from build123d import *

# Parameters (mm, degrees)
EXTRUDE_2_DEPTH                 = 50
SKETCH_4_W                      = 120
SKETCH_4_H                      = 97.901728648
CUT_EXTRUDE_1_DEPTH             = 50
PATTERN_CIRCULAR_1_COUNT        = 8
EXTRUDE_3_DEPTH                 = 50
CUT_EXTRUDE_2_REACH             = 100.489
CUT_EXTRUDE_2_DIRECTION_2_REACH = 100.489
PATTERN_CIRCULAR_3_COUNT        = 8
EXTRUDE_4_DEPTH                 = 50


with BuildPart() as part:
    # Sketch 3 → Extrude 2 (new body)
    with BuildSketch(Plane(origin=(0, 0, 0), x_dir=(1, 0, 0), z_dir=(0, 1, 0))):
        Polygon((-60, 0), (-42.426406871, -42.426406871), (0, -60), (42.426406871, -42.426406871), (60, 0), (42.426406871, 42.426406871), (0, 60), (-42.426406871, 42.426406871), align=None)
        Polygon((-11.480502971, -27.716385975), (11.480502971, -27.716385975), (27.716385975, -11.480502971), (27.716385975, 11.480502971), (11.480502971, 27.716385975), (-11.480502971, 27.716385975), (-27.716385975, 11.480502971), (-27.716385975, -11.480502971), align=None, mode=Mode.SUBTRACT)
    extrude(amount=EXTRUDE_2_DEPTH)

    # Sketch 4 → Cut-Extrude 1 (cut)
    with BuildSketch(Plane(origin=(-16.852857596, 22.400493343, 40.686397374), x_dir=(0.9400294128280147, 0.16450882670917247, 0.2988001823175307), z_dir=(-0.3410933933957357, 0.4533747611963636, 0.8234722963718466))):
        Rectangle(SKETCH_4_W, SKETCH_4_H)
    cut_extrude_1 = extrude(amount=CUT_EXTRUDE_1_DEPTH, mode=Mode.SUBTRACT)

    # Pattern Circular 1: Cut-Extrude 1 ×8 about axis
    pattern_circular_1_axis = Axis((0, 0, 0), (0, 1, 0))
    for i in range(1, PATTERN_CIRCULAR_1_COUNT):
        add(cut_extrude_1.rotate(pattern_circular_1_axis, i * 360 / PATTERN_CIRCULAR_1_COUNT), mode=Mode.SUBTRACT)

    # Sketch 5 → Extrude 3 (add)
    with BuildSketch(Plane(origin=(0, 0, 0), x_dir=(1, 0, 0), z_dir=(0, 1, 0))):
        Polygon((-27.716385975, 11.480502971), (-60, 0), (-27.716385975, -11.480502971), align=None)
    extrude_3 = extrude(amount=EXTRUDE_3_DEPTH)

    # Sketch 6 → Cut-Extrude 2 (cut, up to next)
    with BuildSketch(Plane.XY, mode=Mode.PRIVATE) as cut_extrude_2_sk1:
        Polygon((-27.716385975, 50), (-60, 50), (-60, 25), align=None)
    cut_extrude_2_tool1 = extrude(cut_extrude_2_sk1.sketch, amount=-CUT_EXTRUDE_2_REACH, mode=Mode.PRIVATE) & part.part
    cut_extrude_2 = cut_extrude_2_tool1.solids().sort_by_distance((-49.238795, 41.666667, 0))[0]
    add(cut_extrude_2, mode=Mode.SUBTRACT)

    # Sketch 6 → Cut-Extrude 2 direction 2 (cut, up to next)
    with BuildSketch(Plane.XY, mode=Mode.PRIVATE) as cut_extrude_2_direction_2_sk1:
        Polygon((-27.716385975, 50), (-60, 50), (-60, 25), align=None)
    cut_extrude_2_direction_2_tool1 = extrude(cut_extrude_2_direction_2_sk1.sketch, amount=CUT_EXTRUDE_2_DIRECTION_2_REACH, mode=Mode.PRIVATE) & part.part
    cut_extrude_2_direction_2 = cut_extrude_2_direction_2_tool1.solids().sort_by_distance((-49.238795, 41.666667, 0))[0]
    add(cut_extrude_2_direction_2, mode=Mode.SUBTRACT)

    # Pattern Circular 3: Extrude 3, Cut-Extrude 2, Cut-Extrude 2 direction 2 ×8 about axis
    pattern_circular_3_axis = Axis((0, 0, 0), (0, 1, 0))
    add([extrude_3.rotate(pattern_circular_3_axis, i * 360 / PATTERN_CIRCULAR_3_COUNT) for i in range(1, PATTERN_CIRCULAR_3_COUNT)])
    add([cut_extrude_2.rotate(pattern_circular_3_axis, i * 360 / PATTERN_CIRCULAR_3_COUNT) for i in range(1, PATTERN_CIRCULAR_3_COUNT)], mode=Mode.SUBTRACT)
    add([cut_extrude_2_direction_2.rotate(pattern_circular_3_axis, i * 360 / PATTERN_CIRCULAR_3_COUNT) for i in range(1, PATTERN_CIRCULAR_3_COUNT)], mode=Mode.SUBTRACT)

    # Sketch 3_4 → Extrude 4 (add)
    with BuildSketch(Plane(origin=(0, 0, 0), x_dir=(1, 0, 0), z_dir=(0, 1, 0))):
        Polygon((-27.716385975, -11.480502971), (-11.480502971, -27.716385975), (11.480502971, -27.716385975), (27.716385975, -11.480502971), (27.716385975, 11.480502971), (11.480502971, 27.716385975), (-11.480502971, 27.716385975), (-27.716385975, 11.480502971), align=None)
        Polygon((9.409435159, 22.716385975), (-9.409435159, 22.716385975), (-22.716385975, 9.409435159), (-22.716385975, -9.409435159), (-9.409435159, -22.716385975), (9.409435159, -22.716385975), (22.716385975, -9.409435159), (22.716385975, 9.409435159), align=None, mode=Mode.SUBTRACT)
    extrude(amount=EXTRUDE_4_DEPTH)


solid = part.part
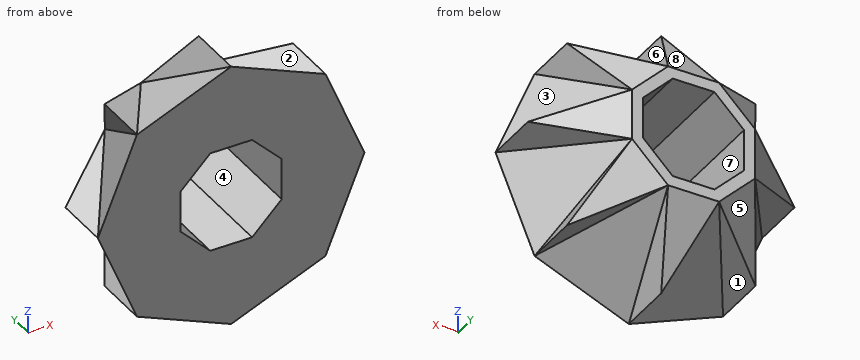
Here's how the part is built. I have some questions about the finished solid (model axes, mm). Face numbers are marked on the shaded views. A direction names the side the tool comes from. Coordinates: 2 decimals unless noted, no trailing zeros. Loops run counter-clockwise (first coordinate to the right, second up) from the corner with the lowest first, then second, coordinate; pieces in that order, holes last.
1. I need wall thicknesses on L1, parallel to X at y = 9, z = -41.5; L2, parallel to Z at x = -22, y = 37.5; L3, parallel to Z at x = 13.5, y = 5. Which ranges of each line are inside material? Lowest first, please.
2. If we mould it in two halves opening along X, with no side actions, what happens to the marked faces 5, 6, 7 and 8? For each: pulls with the +X half, pulls with the -X half, needs draft (parallel to the pull), parting line crosses it, or undercut.
3. For P1, Ø3, axis at x = 45, z = 33, coming from the +Y side; P2, Ø20.5, axis at x = 4.5, y = 34.5, coming from the +Z side; P3, Ø5, axis at y = 24.5, z = -12.5, coming from the +X side, each with a flat end and sliding along its axis, tell me the tip position at first contact or that it passes through.
4. Imagine slicing it at B-B, the plane x = 6.5. Please give me the cut outline in (y, z).
5. For the marked faces 1, 2, 3 and 4, which set-ups out of +Z, -Z, +X, -X, +Y, -Y let a thin tool reach every point of the face, with its end or its side?
6. Imagine slicing it at A-A, the plane z = 6.5. Please give me the cut outline in (x, y), and give its area (3 significant figures).
7. Imagine slicing it at D-D, the plane x = 36. Please give me the cut outline in (y, z).
Taken from the geometry:
1. L1: x = -41.99 to -40.48, -32.7 to 32.7, 40.48 to 41.99
1. L2: z = -32.72 to -10.13, 10.13 to 32.72
1. L3: z = -51.66 to -18.63, 18.63 to 51.66
2. face 5: pulls with the -X half
2. face 6: pulls with the +X half
2. face 7: undercut
2. face 8: needs draft
3. P1: stops at y = 5.37
3. P2: stops at z = 59.69
3. P3: stops at x = 43.06
4. outline: (0, -57.31) - (28.31, -41.72) - (39.15, -41.72) - (50, -27.72) - (50, -22.72) - (0, -22.72) - close; (0, 22.72) - (50, 22.72) - (50, 27.72) - (39.15, 41.72) - (28.31, 41.72) - (0, 57.31) - close
5. face 1: -Z, +Y
5. face 2: +Z, +Y
5. face 3: +X, +Y
5. face 4: +Y, -Y
6. outline: (-57.31, 0) - (-22.72, 0) - (-22.72, 50) - (-27.72, 50) - (-41.72, 39.15) - (-41.72, 28.31) - close; (22.72, 0) - (57.31, 0) - (41.72, 28.31) - (41.72, 39.15) - (27.72, 50) - (22.72, 50) - close
6. area: 2,190 mm2
7. outline: (0, -45.09) - (10.38, -39.37) - (30.19, -39.37) - (35.92, -28.91) - (21.84, -28.91) - (37.17, -8.53) - (43.59, -8.53) - (43.59, 8.53) - (37.17, 8.53) - (21.84, 28.91) - (35.92, 28.91) - (30.19, 39.37) - (10.38, 39.37) - (0, 45.09) - close
